Can you work these out from the model? Positions are in its coordinate system, mm. A direction names the side the tool comes from. Round coordinates to 2 decimals unless told otherwise and drop trailing zeros. Order: outer loops, then holes, each group sorted by start corner. A loop starts at its lowest first (then second) coordinate and runs counter-clockwise, first axis right, second up. Notation, with made-up numbers: (84.25, 66) -> (130.25, 66) arc R20 ccw to (130.25, 75) -> close; hole circle Ø8 at (55, 30). An arc over 180 degrees is marked (long way). One line per item, written item: value.
```python
from build123d import *

# Parameters (mm, degrees)
ESBO_O2_R                = 1.265
RESSALTO_EXTRUS_O1_DEPTH = 5
ESBO_O3_R                = 6.25
CORTE_EXTRUS_O1_DEPTH    = 5
ESBO_O4_R                = 1.265
CORTE_EXTRUS_O2_DEPTH    = 12


with BuildPart() as part:
    # Esboço2 → Ressalto-extrusão1 (new body)
    with BuildSketch(Plane(origin=(0, 0, 0), x_dir=(1, 0, 0), z_dir=(0, 1, 0))):
        with BuildLine():
            Line((0, 0), (37, 0))
            Line((37, 0), (37, 19))
            ThreePointArc((37, 19), (18.5, 37.5), (0, 19))
            Line((0, 19), (0, 0))
        make_face()
        with Locations(Location((10.75, 32.423393759, 0), (0, 0, 270))):
            Circle(ESBO_O2_R, mode=Mode.SUBTRACT)
        with Locations(Location((26.25, 32.423393759, 0), (0, 0, 270))):
            Circle(ESBO_O2_R, mode=Mode.SUBTRACT)
        with Locations(Location((34, 19, 0), (0, 0, 270))):
            Circle(ESBO_O2_R, mode=Mode.SUBTRACT)
        with Locations(Location((26.25, 5.576606241, 0), (0, 0, 270))):
            Circle(ESBO_O2_R, mode=Mode.SUBTRACT)
        with Locations(Location((10.75, 5.576606241, 0), (0, 0, 270))):
            Circle(ESBO_O2_R, mode=Mode.SUBTRACT)
        with Locations(Location((3, 19, 0), (0, 0, 270))):
            Circle(ESBO_O2_R, mode=Mode.SUBTRACT)
    extrude(amount=RESSALTO_EXTRUS_O1_DEPTH)

    # Esboço3 → Corte-extrusão1 (cut)
    with BuildSketch(Plane.XZ):
        with Locations(Location((18.5, -26, 0), (0, 0, 270))):
            Circle(ESBO_O3_R)
    extrude(amount=-CORTE_EXTRUS_O1_DEPTH, mode=Mode.SUBTRACT)

    # Esboço4 → Corte-extrusão2 (cut)
    with BuildSketch(Plane.XY):
        with Locations((3.5, 2.5)):
            Circle(ESBO_O4_R)
        with Locations((18.5, 2.5)):
            Circle(ESBO_O4_R)
        with Locations((33.5, 2.5)):
            Circle(ESBO_O4_R)
    extrude(amount=-CORTE_EXTRUS_O2_DEPTH, mode=Mode.SUBTRACT)


solid = part.part
```
Q1. We'd pull the mould along Z, two halves only. Please class faces 3 (the face through (9.63, 2.46, -4.99)), 4 (the face through (18, 3, -12)), 5 (the face through (17.236, 2.556, -5.916)), 6 (the face through (18.907, 2.465, -37.496)): released by +Z, released by -Z, zero draft, split by the parting line, or undercut.
Answers below:
face 3: undercut
face 4: released by +Z
face 5: zero draft
face 6: released by -Z
Q2. Please list where these lines run through material, in increasing order: line 1 along Z through (x, y) = (27, 3.3); line 2 along X through (y, z) = (3.65, -26); line 3 along Z through (x, y) = (23, 2.2).
Answers below:
line 1: -35.43 to -33.44, -31.4 to -6.6, -4.56 to 0
line 2: 1.38 to 12.25, 24.75 to 35.62
line 3: -36.94 to -30.34, -21.66 to 0
Q3. Will these pins go through, and if not, where does the flat tip stop? pin 1 Ø4 at (x, z) = (26.25, -5.58) entering from -Y; pin 2 Ø0.8 at (x, y) = (34, 3) entering from +Z; pin 3 Ø1.5 at (x, y) = (3.5, 2.5) entering from -Z.
Answers below:
pin 1: y = 0
pin 2: z = -12
pin 3: z = -30.8
Q4. I want a section at C-C on z = -27. List the corners of the cut face in (x, y) for me, plus the area to 3 significant figures.
Answers below:
outline: (1.82, 0) -> (12.33, 0) -> (12.33, 5) -> (1.82, 5) -> close; (24.67, 0) -> (35.18, 0) -> (35.18, 5) -> (24.67, 5) -> close
area: 105 mm^2
Q5. On a 3-axis mill with a long thin cutter (end or side, diameter ignored), from which of +Z, -Z, +X, -X, +Y, -Y can I reach the whole of each face in a straight line? I mean faces 1 (the face through (25.13, 2.46, -4.99)), 2 (the face through (3, 3, -12)). Say none if no direction works.
Answers below:
face 1: +Y, -Y
face 2: +Z
Q6. I want a section at D-D on x = 26.25. List the corners of the cut face in (y, z) for me, plus the area to 3 significant figures.
Answers below:
outline: (0, -35.8) -> (5, -35.8) -> (5, -33.69) -> (0, -33.69) -> close; (0, -31.16) -> (5, -31.16) -> (5, -6.84) -> (0, -6.84) -> close; (0, -4.31) -> (5, -4.31) -> (5, 0) -> (0, 0) -> close
area: 154 mm^2
Q7. I want a section at A-A on x = 18.5. List the corners of the cut face in (y, z) for me (3 decimals).
Answers below:
outline: (0, -37.5) -> (5, -37.5) -> (5, -32.25) -> (0, -32.25) -> close; (0, -19.75) -> (5, -19.75) -> (5, 0) -> (3.765, 0) -> (3.765, -12) -> (1.235, -12) -> (1.235, 0) -> (0, 0) -> close
Q8. I want a section at B-B on z = -2.5. List the corners of the cut face in (x, y) for me (3 decimals), plus the area to 3 significant figures.
Answers below:
outline: (0, 0) -> (37, 0) -> (37, 5) -> (0, 5) -> close; hole circle Ø2.53 at (3.5, 2.5); hole circle Ø2.53 at (18.5, 2.5); hole circle Ø2.53 at (33.5, 2.5)
area: 170 mm^2
